from build123d import *

# Parameters (mm, degrees)
SKETCH4_R           = 6.45
BOSS_EXTRUDE3_DEPTH = 3.1
SKETCH5_R           = 2
SKETCH5_R_2         = 3
CUT_EXTRUDE4_DEPTH  = 4.1
FILLET1_R           = 10
SKETCH6_W           = 50
SKETCH6_H           = 3.1
BOSS_EXTRUDE4_DEPTH = 3.1
CHAMFER1_SIZE       = 15
FILLET2_R           = 10


with BuildPart() as part:
    # Sketch4 → Boss-Extrude3 (new body)
    with BuildSketch(Plane.XY):
        Polygon((50.399999987, -5.000794186), (-50.399999987, -5.000794186), (-50.399999987, 44.999205814), (-0.399999987, 44.999205814), (19.600000013, 44.999205814), (50.399999987, 44.999205814), align=None)
        with Locations((12.5, 5.000000001)):
            Circle(SKETCH4_R, mode=Mode.SUBTRACT)
        with Locations((-37.499999987, 4.999205814)):
            Circle(SKETCH4_R, mode=Mode.SUBTRACT)
        with Locations((37.499999987, 4.999205814)):
            Circle(SKETCH4_R, mode=Mode.SUBTRACT)
        with Locations((-12.5, 5.000000001)):
            Circle(SKETCH4_R, mode=Mode.SUBTRACT)
    extrude(amount=BOSS_EXTRUDE3_DEPTH)

    # Sketch5 → Cut-Extrude4 (cut, through all)
    with BuildSketch(Plane.XY):
        with Locations((22.35, 35.250000001)):
            Circle(SKETCH5_R)
        with Locations((22.35, 25.250000001)):
            Circle(SKETCH5_R)
        with Locations((-26.65, 25.250000001)):
            Circle(SKETCH5_R)
        with Locations((-26.65, 35.250000001)):
            Circle(SKETCH5_R)
        with Locations((37.5, 24.999205814)):
            Circle(SKETCH5_R_2)
        with Locations((-37.5, 24.999205814)):
            Circle(SKETCH5_R_2)
        with BuildLine():
            Line((-22.5, 20.000000001), (18.2, 20.000000001))
            Line((18.2, 20.000000001), (18.2, 40.500000001))
            Line((18.2, 40.500000001), (-22.5, 40.500000001))
            Line((-22.5, 40.500000001), (-22.5, 33.250000001))
            add(Edge.make_bspline(
                [(-28.5, 30.250000001), (-28.211982464, 32.604979652), (-24.313004512, 33.611534185), (-22.5, 33.250000001)],
                knots=[0, 0, 0, 0, 1, 1, 1, 1], degree=3))
            add(Edge.make_bspline(
                [(-28.5, 30.250000001), (-28.211982464, 27.89502035), (-24.313004512, 26.888465817), (-22.5, 27.250000001)],
                knots=[0, 0, 0, 0, 1, 1, 1, 1], degree=3))
            Line((-22.5, 27.250000001), (-22.5, 20.000000001))
        make_face()
    extrude(amount=CUT_EXTRUDE4_DEPTH, mode=Mode.SUBTRACT)

    # Fillet1
    fillet1_edges = [part.edges().sort_by_distance(p)[0] for p in [
        (50.399999987, -5.000794186, 1.55),
        (-50.399999987, -5.000794186, 1.55),
    ]]
    fillet(fillet1_edges, radius=FILLET1_R)

    # Sketch6 → Boss-Extrude4 (add, through all)
    with BuildSketch(Plane.XY.offset(3.1)):
        with Locations((0, 46.549205814)):
            Rectangle(SKETCH6_W, SKETCH6_H)
    extrude(amount=-BOSS_EXTRUDE4_DEPTH)

    # Chamfer1
    chamfer1_edges = [part.edges().sort_by_distance(p)[0] for p in [
        (50.399999987, 44.999205814, 1.55),
        (-50.399999987, 44.999205814, 1.55),
    ]]
    chamfer(chamfer1_edges, length=CHAMFER1_SIZE)

    # Fillet2
    fillet2_edges = [part.edges().sort_by_distance(p)[0] for p in [
        (-50.399999987, 29.999205814, 1.55),
        (50.399999987, 29.999205814, 1.55),
    ]]
    fillet(fillet2_edges, radius=FILLET2_R)


solid = part.part
Here's how the part is built. I have some questions about the finished solid (model axes, mm). A direction names the side the tool comes from. Give positions to 0.01 mm unless a question says otherwise; leave off trailing zeros. Order: outer loops, then holes, each group sorted by start corner. A loop starts at its lowest first (then second) coordinate and runs counter-clockwise, first axis right, second up. Notation, with made-up numbers: M 7,54 L 16,54 A19 ccw 16,87 Z; hole C -4,-19 d5. An arc over 180 degrees is marked long. Answer as a JSON object with one key per item and string values. Group by question number.
1) Suppose I cut it at A-A, the plane x = 22.35. Write out the boundary of the cut face in (y, z), plus the area to 3 significant figures.
2) We'd pull the mould along X, two halves only. Please class faces 4 (the cylindrical face through (18.65, 6.94, 1.53)), 5 (the flat face through (25, 47, 2)), 6 (the cylindrical face through (-47.39, -2.15, 1.57)): pulls with the +X half, pulls with the -X half, needs draft (parallel to the pull), parting line crosses it, or undercut.
3) On a 3-axis mill with a long thin cutter (end or side, diameter ignored), from which of +Z, -Z, +X, -X, +Y, -Y can I reach the whole of each face in a straight line? I mean faces 1 (the flat face through (50.4, 16, 2)), 2 (the flat face through (-25, 47, 2)), 3 (the flat face through (-22.5, 24, 2)). Say none if no direction works.
4) Suppose I cut it at B-B, the plane x = -41.5. Write out the boundary of the cut face in (y, z), plus the area to 3 significant figures.
5) I'm going to push flat-ended pins straight in: pin 1 Ø20.5 at (x, y) = (37.5, 5) entering from +Z; pin 2 Ø1.6 at (y, z) = (36.5, 1.5) entering from +X; pin 3 Ø1.6 at (x, z) = (30.5, 1.5) entering from +Y; pin 4 Ø0.9 at (y, z) = (29.5, 1) entering from -X. Where does each tip first touch, or does it pass through?
6) Please list where these lines run through material, in increasing order: L1, parallel to Y at x = 12.5, z = 1.1; L2, parallel to X at y = 40, z = 2.45; L3, parallel to X at y = 22.5, z = 2.95. Write a range as [from, to].
7) Suppose I cut it at C-C, the plane y = 35.25. Write out the boundary of the cut face in (x, z).
8) Suppose I cut it at D-D, the plane x = -15. Write out the boundary of the cut face in (y, z), plus the area to 3 significant figures.
Results found:
{
 "1": {"outline": "M -5,0 L 23.25,0 L 23.25,3.1 L -5,3.1 Z; M 27.25,0 L 33.25,0 L 33.25,3.1 L 27.25,3.1 Z; M 37.25,0 L 48.1,0 L 48.1,3.1 L 37.25,3.1 Z", "area": "140 mm²"},
 "2": {"face 4": "undercut", "face 5": "pulls with the +X half", "face 6": "pulls with the -X half"},
 "3": {"face 1": "+Z, -Z, +X, +Y, -Y", "face 2": "+Z, -Z, -X, +Y", "face 3": "+Z, -Z"},
 "4": {"outline": "M -4.94,0 L -0.06,0 L -0.06,3.1 L -4.94,3.1 Z; M 10.06,0 L 38.9,0 L 38.9,3.1 L 10.06,3.1 Z", "area": "105 mm²"},
 "5": {"pin 1": "z = 3.1", "pin 2": "x = 44.7", "pin 3": "y = 45", "pin 4": "x = -49.88"},
 "6": {"L1": "[-5, -1.45], [11.45, 20], [40.5, 48.1]", "L2": "[-40.4, -22.5], [18.2, 40.4]", "L3": "[-50.4, -39.16], [-35.84, -22.5], [18.2, 35.84], [39.16, 50.4]"},
 "7": {"outline": "M -45.15,0 L -28.65,0 L -28.65,3.1 L -45.15,3.1 Z; M -24.65,0 L -22.5,0 L -22.5,3.1 L -24.65,3.1 Z; M 18.2,0 L 20.35,0 L 20.35,3.1 L 18.2,3.1 Z; M 24.35,0 L 45.15,0 L 45.15,3.1 L 24.35,3.1 Z"},
 "8": {"outline": "M -5,0 L -0.95,0 L -0.95,3.1 L -5,3.1 Z; M 10.95,0 L 20,0 L 20,3.1 L 10.95,3.1 Z; M 40.5,0 L 48.1,0 L 48.1,3.1 L 40.5,3.1 Z", "area": "64.2 mm²"}
}
